The listing builds one solid part. Answer for the finished solid, in the listing's coordinates (mm). A direction names the side the tool comes from. Round coordinates to 2 decimals unless told otherwise and drop trailing zeros. Write each loop counter-clockwise with the first axis right and the second up, starting at its lowest first coordinate (ties: lowest second). Pieces come first, ordered by that corner, then holes. Notation, with made-up numbers: M 62.5,-9 L 100.5,-9 A30 cw 100.5,17 Z; hole C 79.25,-0.75 d4. An arc over 180 degrees is marked long. One line per item, written item: value. Start each with the question number.
(1) Section B-B (y = -76) is taken. Determine the outline of the cut face in (x, z).
(2) Consider probe 1 along X at (y, z) = (-40, 0.65); probe 2 along Y at (x, z) = (72.39, 1.3); probe 3 along Y at (x, z) = (107.5, 2.9). Determine where each line is inside the solid, lowest interval first.
(3) For faces 5 (the flat face through (112, -82.404, 3)), 6 (the flat face through (112, -63.354, 3)), 7 (the flat face through (3, -63.354, 3)), 8 (the flat face through (67.564, -40, 3)), 9 (the flat face through (5.08, -93, 3)), determine the directions among +Z, -Z, +X, -X, +Y, -Y from which every point of the face is accessible in a straight line to the end or side of a thin tool.
(4) Section D-D (y = -50) is taken. Determine the outline of the cut face in (x, z), plus the area to 3 significant figures.
(5) Given P1, Ø2.5, axis at y = -39.5, z = 3.5, coming from the +X side; P2, Ø2.5, axis at x = 112, z = 4, coming from the -Y side; P3, Ø2.5, axis at y = -40.5, z = 3, coming from the -X side, each flat-ended and moving along its own axis, determine where each tip first touches the part or whether it passes through.
(6) Section C-C (z = 4.35) is taken. Determine the outline of the cut face in (x, y), plus the area to 3 significant figures.
(7) For a pull along X with two mould halves and no side action, classify faces 1 (the flat face through (109.22, -93, 3)), 2 (the cylindrical face through (26.233, -68.667, 2.755)), 3 (the flat face through (5.08, -53, 3)), 4 (the flat face through (78, -37.319, 3)) as released by +X, released by -X, zero draft, split by the parting line, or undercut.
(8) Section A-A (x = 72.39) is taken. Determine the outline of the cut face in (y, z).
```python
from build123d import *

# Parameters (mm, degrees)
SKETCH1_R           = 2.489200007
SKETCH1_R_2         = 3.225800007
SKETCH1_R_3         = 12.801600005
BOSS_EXTRUDE1_DEPTH = 5.588


with BuildPart() as part:
    # Sketch1 → Boss-Extrude1 (new body)
    with BuildSketch(Plane.XY):
        Polygon((5.08, -82.404335154), (5.08, -103.359335154), (109.22, -103.359335154), (109.22, -82.404335154), (114.3, -82.404335154), (114.3, -63.354335154), (109.22, -63.354335154), (109.22, -42.399335154), (88.392, -42.399335154), (88.392, -37.319335154), (67.564, -37.319335154), (67.564, -42.399335154), (46.736, -42.399335154), (46.736, -37.319335154), (25.908, -37.319335154), (25.908, -42.399335154), (5.08, -42.399335154), (5.08, -63.354335154), (0, -63.354335154), (0, -82.404335154), align=None)
        with Locations((26.772733885, -66.237193374)):
            Circle(SKETCH1_R, mode=Mode.SUBTRACT)
        with Locations((37.089955672, -71.097217628)):
            Circle(SKETCH1_R_2, mode=Mode.SUBTRACT)
        with Locations((72.39, -87.725635154)):
            Circle(SKETCH1_R_3, mode=Mode.SUBTRACT)
    extrude(amount=BOSS_EXTRUDE1_DEPTH)


solid = part.part
```
Recorded:
1. outline: M 0,0 L 67.25,0 L 67.25,5.59 L 0,5.59 Z; M 77.53,0 L 114.3,0 L 114.3,5.59 L 77.53,5.59 Z
2. probe 1: x = 25.91 to 46.74, 67.56 to 88.39
2. probe 2: y = -103.36 to -100.53, -74.92 to -37.32
2. probe 3: y = -103.36 to -42.4
3. face 5: +Z, -Z, +X, -Y
3. face 6: +Z, -Z, +X, +Y
3. face 7: +Z, -Z, -X, +Y
3. face 8: +Z, -Z, +Y
3. face 9: +Z, -Z, -X, -Y
4. outline: M 5.08,0 L 109.22,0 L 109.22,5.59 L 5.08,5.59 Z
4. area: 582 mm2
5. P1: stops at x = 88.39
5. P2: stops at y = -82.4
5. P3: stops at x = 25.91
6. outline: M 0,-82.4 L 5.08,-82.4 L 5.08,-103.36 L 109.22,-103.36 L 109.22,-82.4 L 114.3,-82.4 L 114.3,-63.35 L 109.22,-63.35 L 109.22,-42.4 L 88.39,-42.4 L 88.39,-37.32 L 67.56,-37.32 L 67.56,-42.4 L 46.74,-42.4 L 46.74,-37.32 L 25.91,-37.32 L 25.91,-42.4 L 5.08,-42.4 L 5.08,-63.35 L 0,-63.35 Z; hole C 26.77,-66.24 d4.98; hole C 37.09,-71.1 d6.45; hole C 72.39,-87.73 d25.6
6. area: 6,190 mm2
7. face 1: released by +X
7. face 2: undercut
7. face 3: released by -X
7. face 4: zero draft
8. outline: M -103.36,0 L -100.53,0 L -100.53,5.59 L -103.36,5.59 Z; M -74.92,0 L -37.32,0 L -37.32,5.59 L -74.92,5.59 Z
